```python
from build123d import *

# Parameters (mm, degrees)
SKETCH1_R           = 12.4
MAIN_EXTRUDE_DEPTH  = 64.7
SKETCH2_R           = 3.5
BOSS_EXTRUDE2_DEPTH = 2.4
SKETCH3_R           = 2
BOSS_EXTRUDE3_DEPTH = 9.6
KEY_CUT_DEPTH       = 8


with BuildPart() as part:
    # Sketch1 → Main Extrude (new body)
    with BuildSketch(Plane.XY):
        Circle(SKETCH1_R)
    extrude(amount=MAIN_EXTRUDE_DEPTH)

    # Sketch2 → Boss-Extrude2 (add)
    with BuildSketch(Plane.XY.offset(64.7)):
        Circle(SKETCH2_R)
    extrude(amount=BOSS_EXTRUDE2_DEPTH)

    # Sketch3 → Boss-Extrude3 (add)
    with BuildSketch(Plane.XY.offset(67.1)):
        Circle(SKETCH3_R)
    extrude(amount=BOSS_EXTRUDE3_DEPTH)

    # Sketch5 → Key Cut (cut)
    with BuildSketch(Plane.XY.offset(76.7)):
        with BuildLine():
            Line((-1.472086844, 1.353868651), (1.472086844, 1.353868651))
            ThreePointArc((1.472086844, 1.353868651), (0, 2), (-1.472086844, 1.353868651))
        make_face()
    extrude(amount=-KEY_CUT_DEPTH, mode=Mode.SUBTRACT)


solid = part.part
```
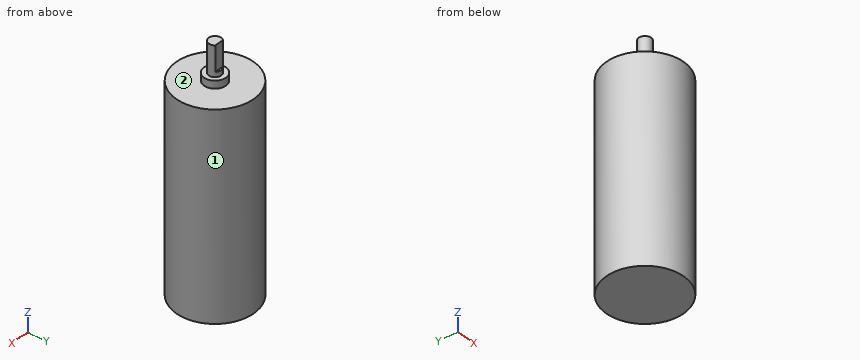
Work out the finished part from the listing and answer in its coordinate system (mm). Face numbers are marked on the shaded views. A direction names the side the tool comes from. Give positions to 0.01 mm unless a question says otherwise; leave off trailing zeros. Loops run counter-clockwise (first coordinate to the right, second up) from the corner with the lowest first, then second, coordinate; pieces in that order, holes last. Notation, with made-up numbers: (35, -16) -> (51, -16) arc R6 ccw to (51, -9) -> close; hole circle Ø7 at (-14.75, 2). An arc over 180 degrees is marked (long way). Put each result on its own line as item: value. Start each with the question number.
Item 1: The part is cut by section A-A (x = 0). Give the vertices of the cut face in (y, z).
Item 2: The part is cut by section D-D (z = 71.5). Give the vertices of the cut face in (x, y).
Item 3: Each of these flat-tipped pins is pushed along its axis until it touches: P1, Ø3, axis at x = 6, y = 4.5, coming from the +Z side; P2, Ø4, axis at x = -6.5, z = 67.5, coming from the -Y side; P3, Ø1.5, axis at x = 0, z = 74, coming from the +Y side; P4, Ø12, axis at y = 10, z = 43.5, coming from the -X side. Where does it stop, or does it pass through?
Item 4: Which of the six approach directions +Z, -Z, +X, -X, +Y, -Y give full straight-line access (tool end or side, diameter ignored) to the marked faces 1 and 2?
Item 5: The part is cut by section C-C (z = 26.5). Give the vertices of the cut face in (x, y), then the cut area to 3 significant figures.
Item 6: The part is cut by section B-B (y = 0). Give the vertices of the cut face in (x, z), then the cut area to 3 significant figures.
Item 7: Find the intervals of material crossed by L1, parallel to Z at x = -11, y = -5; L2, parallel to Y at x = 0.5, z = 59.5, in increasing order. Write a range as [from, to].
Answers below:
1. outline: (-12.4, 0) -> (12.4, 0) -> (12.4, 64.7) -> (3.5, 64.7) -> (3.5, 67.1) -> (2, 67.1) -> (2, 68.7) -> (1.35, 68.7) -> (1.35, 76.7) -> (-2, 76.7) -> (-2, 67.1) -> (-3.5, 67.1) -> (-3.5, 64.7) -> (-12.4, 64.7) -> close
2. outline: (-1.47, 1.35) arc R2 ccw (long way) to (1.47, 1.35) -> close
3. P1: z = 64.7
3. P2: through
3. P3: y = 1.35
3. P4: x = -11.74
4. face 1: +Z, -Z
4. face 2: +Z
5. outline: circle Ø24.8 at (0, 0)
5. area: 483 mm2
6. outline: (-12.4, 0) -> (12.4, 0) -> (12.4, 64.7) -> (3.5, 64.7) -> (3.5, 67.1) -> (2, 67.1) -> (2, 76.7) -> (-2, 76.7) -> (-2, 67.1) -> (-3.5, 67.1) -> (-3.5, 64.7) -> (-12.4, 64.7) -> close
6. area: 1,660 mm2
7. L1: [0, 64.7]
7. L2: [-12.39, 12.39]
